Could you check a few things on this model? Use its own coordinates, in mm. Face numbers are marked on the shaded views. A direction names the side the tool comes from. Give positions to 0.01 mm unless a question says otherwise; leave off trailing zeros. Order: outer loops, then holes, each group sorted by start corner. A loop starts at its lowest first (then second) coordinate and runs counter-clockwise, first axis right, second up. Notation, with made-up numbers: M 47.5,64.25 L 56.5,64.25 A10 cw 56.5,70.25 Z; hole C -19.5,6.5 d11. An arc over 180 degrees is marked long. Use a Markdown table: item, result. Add a question column.
```python
from build123d import *

# Parameters (mm, degrees)
F0_W     = 57.15
F0_H     = 44.45
F1_DEPTH = 25.4
F3_DEPTH = 12.7
F5_DEPTH = 25.4


with BuildPart() as f1:
    # F0 (on Front) → F1 (new body)
    with BuildSketch(Plane.XZ):
        with Locations((8.218082, 9.456021)):
            Rectangle(F0_W, F0_H)
    extrude(amount=F1_DEPTH)

    # F2 (on face) → F3 (cut)
    with BuildSketch(Plane.XZ.offset(25.4)):
        Polygon((36.793082, 31.681021), (-1.306918, 31.681021), (24.093082, -12.768979), (36.793082, -12.768979), align=None)
    extrude(amount=-F3_DEPTH, mode=Mode.SUBTRACT)

    # F4 (on face) → F5 (cut)
    with BuildSketch(Plane.XZ.offset(25.4)):
        with BuildLine():
            Line((3.277831, 23.657709), (9.578796, 12.631021))
            Line((9.578796, 12.631021), (22.278796, 12.631021))
            ThreePointArc((22.278796, 12.631021), (15.953267, 23.61538), (3.277831, 23.657709))
        make_face()
        with BuildLine():
            Line((9.578796, 12.631021), (-3.121204, 12.631021))
            ThreePointArc((-3.121204, 12.631021), (3.204325, 1.646663), (15.87976, 1.604333))
            Line((15.87976, 1.604333), (9.578796, 12.631021))
        make_face()
        with BuildLine():
            Line((9.578796, 12.631021), (15.87976, 1.604333))
            ThreePointArc((15.87976, 1.604333), (20.563154, 6.256551), (22.278796, 12.631021))
            Line((22.278796, 12.631021), (9.578796, 12.631021))
        make_face()
        with BuildLine():
            ThreePointArc((3.277831, 23.657709), (-1.405562, 19.005492), (-3.121204, 12.631021))
            Line((-3.121204, 12.631021), (9.578796, 12.631021))
            Line((9.578796, 12.631021), (3.277831, 23.657709))
        make_face()
    extrude(amount=-F5_DEPTH, mode=Mode.SUBTRACT)


solid = f1.part
```
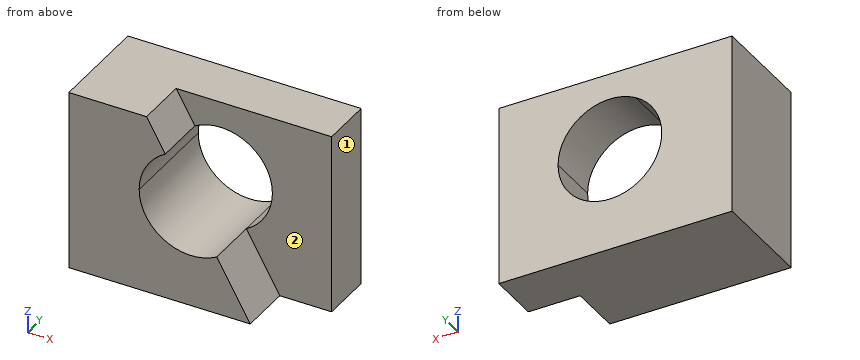
1) Suppose I cut it at A-A on x = 13. Please give me the cut outline in (y, z).
2) Suppose I cut it at C-C on z = 21.5. Please give me the cut outline in (x, y).
3) Please list where these lines run through material, in increasing order: line 1 (Z direction, x = 10, y = -5); line 2 (Y direction, x = 23, z = 10); line 3 (X direction, y = -11, z = 17). Write a range as from..to.
4) For the marked faces 1 and 2, which set-ups out of +Z, -Z, +X, -X, +Y, -Y let a thin tool reach every point of the face, with its end or its side?
5) For pin 1 (8 mm diameter, centred on x = 16, z = 24.5, fed in from -Y); pin 2 (1.5 mm diameter, centred on y = -18, z = 6, fed in from +X), each with a flat end and sliding along its axis, tell me the tip position at first contact or that it passes through.
6) Suppose I cut it at B-B on y = -2.5. Please give me the cut outline in (x, z), and give its area (3 significant figures).
Values found:
| question | item | result |
|---|---|---|
| 1 | outline | M -25.4,-12.77 L 0,-12.77 L 0,0.4 L -25.4,0.4 Z; M -12.7,24.86 L 0,24.86 L 0,31.68 L -12.7,31.68 Z |
| 2 | outline | M -20.36,-25.4 L 0.49,-25.4 L 0.49,0 L -20.36,0 Z; M 18.67,-12.7 L 36.79,-12.7 L 36.79,0 L 18.67,0 Z |
| 3 | line 1 | z = -12.77..-0.06, 25.32..31.68 |
| 3 | line 2 | y = -12.7..0 |
| 3 | line 3 | x = -20.36..-2.35, 21.5..36.79 |
| 4 | face 1 | +Z, -Z, +X, +Y, -Y |
| 4 | face 2 | +Z, +X, -Y |
| 5 | pin 1 | stops at y = -12.7 |
| 5 | pin 2 | stops at x = -0.76 |
| 6 | outline | M -20.36,-12.77 L 36.79,-12.77 L 36.79,31.68 L -20.36,31.68 Z; hole M -3.12,12.63 A12.7 ccw 15.88,1.6 A12.7 ccw 22.28,12.63 A12.7 ccw 3.28,23.66 A12.7 ccw Z |
| 6 | area | 2,030 mm^2 |
